The figure shows three views and two pictorial views of one solid part (mm, origin at its lowest corner). Answer the questions. A direction names the side the tool comes from. Give positions to 0.01 mm unless a question says otherwise; leave off trailing zeros. Write each loop counter-clockwise with the first axis right and the second up, starting at its lowest first coordinate (ties: lowest second). Pieces come first, ordered by that corner, then holes. Notation, with made-up numbers: (42.5, 79.5) -> (86.5, 79.5) arc R15 cw to (86.5, 96.5) -> close; hole circle Ø3 at (85.25, 11). An arc over 180 degrees is marked (long way). Answer as CSV lines item,"result". Start each with the question number.
1. The part is cut by section C-C, the plane y = 10. Determine the outline of the cut face in (x, z), and give its area (4 significant figures).
2. The part is cut by section D-D, the plane z = 41.5. Determine the outline of the cut face in (x, y), and give its area (3 significant figures).
3. The part is cut by section B-B, the plane y = 2.5. Determine the outline of the cut face in (x, z).
4. The part is cut by section A-A, the plane z = 29. Determine the outline of the cut face in (x, y), and give its area (3 significant figures).
5. A tool of negligible diameter and unlimited length cuts with its end or side. For the marked faces 4, 5, 6, 7 and 8, from which of +Z, -Z, +X, -X, +Y, -Y can it reach the whole face along a straight path? Write none if from no direction.
6. For a pull along X with two mould halves and no side action, classify the marked faces 1, 2 and 3 as pulls with the +X half, pulls with the -X half, needs draft (parallel to the pull), parting line crosses it, or undercut.
7. Given pin 1 (1.5 mm diameter, centred on x = 8.5, y = 2.5, fed in from -Z); pin 2 (4.5 mm diameter, centred on y = 1.5, z = 4, fed in from +X); pin 3 (1.5 mm diameter, centred on x = 33, z = 26, fed in from -Y), each flat-ended and moving along its own axis, determine where each tip first touches the part or whether it passes through.
8. Find the intervals of material crossed by line 1 (Z direction, x = 9.25, y = 2.5); line 2 (Z direction, x = 6.5, y = 17.5); line 3 (Z direction, x = 9, y = 19.5), in increasing order.
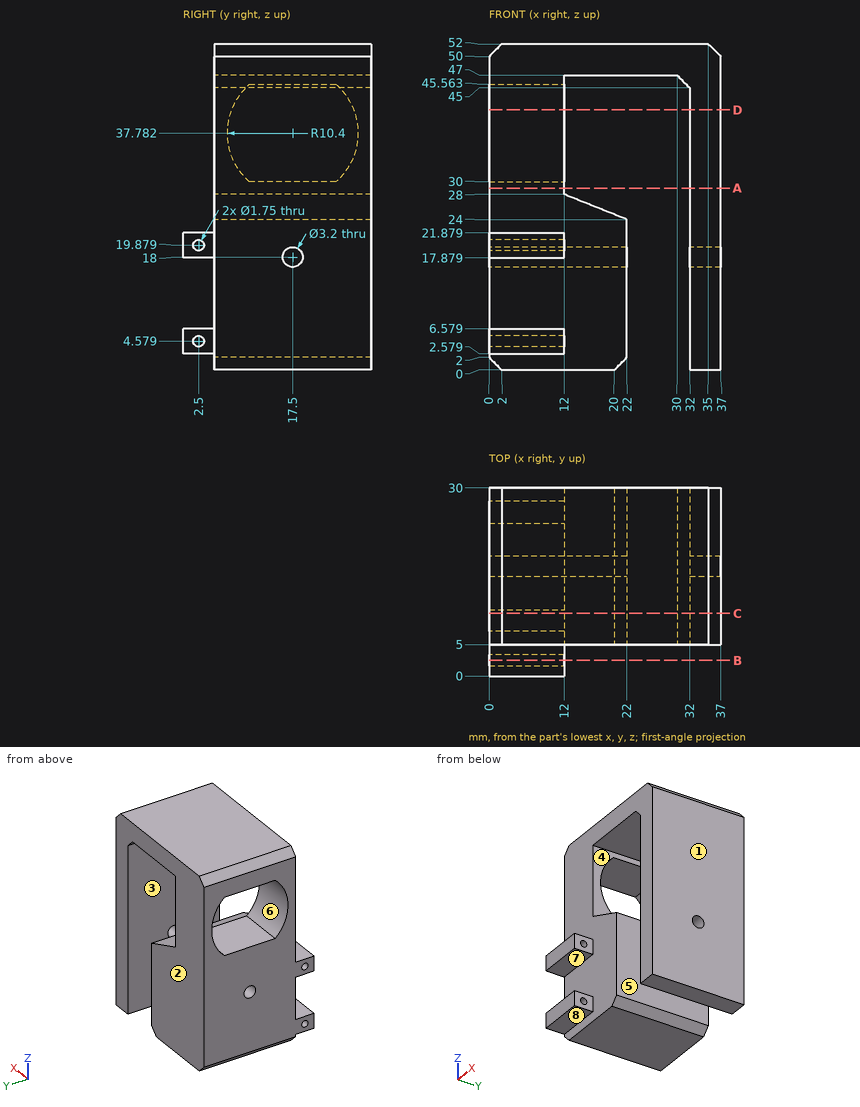
Results found:
1,outline,"(0, 2) -> (2, 0) -> (20, 0) -> (22, 2) -> (22, 24) -> (12, 28) -> (12, 30.58) -> (0, 30.58) -> close; (0, 44.99) -> (12, 44.99) -> (12, 47) -> (30, 47) -> (32, 45) -> (32, 0) -> (37, 0) -> (37, 50) -> (35, 52) -> (2, 52) -> (0, 50) -> close"
1,area,"1,065 mm²"
2,outline,"(0, 5) -> (12, 5) -> (12, 7.79) -> (0, 7.79) -> close; (0, 27.21) -> (12, 27.21) -> (12, 30) -> (0, 30) -> close; (32, 5) -> (37, 5) -> (37, 30) -> (32, 30) -> close"
2,area,"192 mm²"
3,outline,"(0, 2.58) -> (12, 2.58) -> (12, 3.7) -> (0, 3.7) -> close; (0, 5.45) -> (12, 5.45) -> (12, 6.58) -> (0, 6.58) -> close; (0, 17.88) -> (12, 17.88) -> (12, 19) -> (0, 19) -> close; (0, 20.75) -> (12, 20.75) -> (12, 21.88) -> (0, 21.88) -> close"
4,outline,"(0, 5) -> (12, 5) -> (12, 30) -> (0, 30) -> close; (32, 5) -> (37, 5) -> (37, 30) -> (32, 30) -> close"
4,area,"425 mm²"
5,face 4,"+Y, -Y"
5,face 5,"-Z, +Y, -Y"
5,face 6,"-X"
5,face 7,"+X, -X, -Y"
5,face 8,"-Z, +X, -X, -Y"
6,face 1,"pulls with the +X half"
6,face 2,"needs draft"
6,face 3,"undercut"
7,pin 1,"stops at z = 2.58"
7,pin 2,"stops at x = 12"
7,pin 3,"stops at y = 5"
8,line 1,"z = 2.58 to 3.7, 5.45 to 6.58, 17.88 to 19, 20.75 to 21.88"
8,line 2,"z = 0 to 16.4, 19.6 to 30, 45.56 to 52"
8,line 3,"z = 0 to 30, 45.56 to 52"
